Source: CAD feature listing. Evaluate the final solid. Frame: model axes, mm. Face numbers are marked on the shaded views. A direction names the side the tool comes from. Coordinates: 2 decimals unless noted, no trailing zeros. Order: outer loops, then holes, each group sorted by start corner. A loop starts at its lowest first (then second) coordinate and runs counter-clockwise, first axis right, second up. Notation, with made-up numbers: (67.5, -12.5) -> (105.5, -12.5) arc R25 cw to (105.5, -0.5) -> close; hole circle Ø8 at (26, -15.5). An arc over 180 degrees is marked (long way). Write item = value, one per line. Start each with the question number.
Item 1: Ray query, line 1 along Y through (x, z) = (-35, 22.25); line 2 along X through (y, z) = (20, 5.5); line 3 along X through (y, z) = (0, 11). Return the intervals inside material, ascending. Write a range as [from, to].
Item 2: Section query A-A (y = 0). Output: boundary loops of the cut face in (x, z), then the cut area to 3 significant figures.
Item 3: Contact query for flat-ended pins moving along their axis: pin 1 (1.5 mm diameter, centred on y = -18, z = 11.5, fed in from +X); pin 2 (3 mm diameter, centred on x = -39.5, z = 21.5, fed in from +Y); pin 3 (4 mm diameter, centred on x = -36.5, y = 28, fed in from -Z); pin 4 (2 mm diameter, centred on x = 32, z = 16, fed in from -Y). Output: stop coordinate, or through.
Item 4: Set-up query: the marked faces 1, 2 and 3. Return all of +Z, -Z, +X, -X, +Y, -Y with unobstructed straight access to the full face (end or side cutting, diameter ignored); none if empty.
Item 5: Section query C-C (y = -29). Output: boundary loops of the cut face in (x, z), then the cut area to 3 significant figures.
Item 6: Mould query, pull axis X, two halves, no side actions, for the marked faces 4, 5 and 6. Classes: released by +X, released by -X, zero draft, split by the parting line, or undercut.
Item 7: Section query B-B (y = -44). Output: boundary loops of the cut face in (x, z), then the cut area to 3 significant figures.
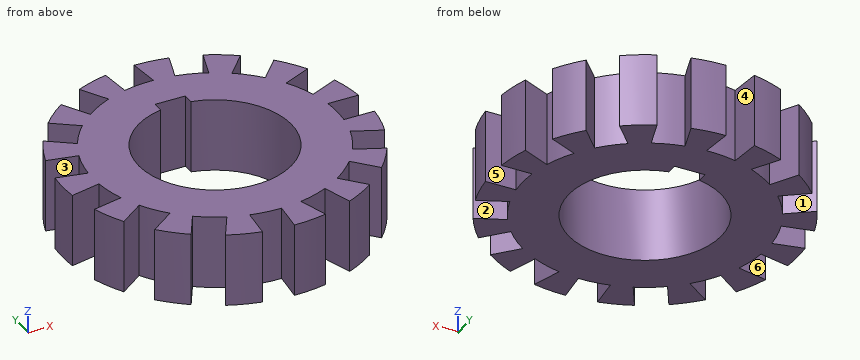
```python
from build123d import *

# Parameters (mm, degrees)
BOSS_EXTRUDE2_DEPTH = 24


with BuildPart() as part:
    # Sketch1 → Boss-Extrude2 (new body)
    with BuildSketch(Plane.XY):
        with BuildLine():
            Line((39.686269666, 5), (49.749371855, 5))
            ThreePointArc((49.749371855, 5), (48.907380037, 10.395584541), (47.481995894, 15.667165215))
            Line((47.481995894, 15.667165215), (38.2888946, 11.574132812))
            ThreePointArc((38.2888946, 11.574132812), (36.541818306, 16.269465723), (34.221528169, 20.709587388))
            Line((34.221528169, 20.709587388), (43.414629464, 24.802619792))
            ThreePointArc((43.414629464, 24.802619792), (40.450849719, 29.389262615), (37.004551483, 33.625335233))
            Line((37.004551483, 33.625335233), (30.271021813, 26.146992913))
            ThreePointArc((30.271021813, 26.146992913), (26.765224254, 29.725793019), (22.839573558, 32.838298977))
            Line((22.839573558, 32.838298977), (29.573103228, 40.316641297))
            ThreePointArc((29.573103228, 40.316641297), (25, 43.301270189), (20.128683944, 45.769379313))
            Line((20.128683944, 45.769379313), (17.019014352, 36.198800401))
            ThreePointArc((17.019014352, 36.198800401), (12.360679775, 38.042260652), (7.508449189, 39.288970345))
            Line((7.508449189, 39.288970345), (10.618118781, 48.859549256))
            ThreePointArc((10.618118781, 48.859549256), (5.226423163, 49.726094768), (-0.227615912, 49.999481907))
            Line((-0.227615912, 49.999481907), (0.824264696, 39.991506445))
            ThreePointArc((0.824264696, 39.991506445), (-4.181138531, 39.780875815), (-9.120954258, 38.946221812))
            Line((-9.120954258, 38.946221812), (-10.172834865, 48.954197275))
            ThreePointArc((-10.172834865, 48.954197275), (-15.450849719, 47.552825815), (-20.544558909, 45.584219849))
            Line((-20.544558909, 45.584219849), (-15.513007814, 36.869317712))
            ThreePointArc((-15.513007814, 36.869317712), (-20, 34.641016151), (-24.173261852, 31.869317712))
            Line((-24.173261852, 31.869317712), (-29.204812947, 40.584219849))
            ThreePointArc((-29.204812947, 40.584219849), (-33.456530318, 37.157241274), (-37.309161029, 33.287032059))
            Line((-37.309161029, 33.287032059), (-29.167940342, 27.372089))
            ThreePointArc((-29.167940342, 27.372089), (-32.360679775, 23.511410092), (-35.045792865, 19.281919056))
            Line((-35.045792865, 19.281919056), (-43.187013552, 25.196862116))
            ThreePointArc((-43.187013552, 25.196862116), (-45.677272882, 20.336832154), (-47.622670264, 15.234214023))
            Line((-47.622670264, 15.234214023), (-37.779471002, 13.141977432))
            ThreePointArc((-37.779471002, 13.141977432), (-39.125904029, 8.316467633), (-39.85858791, 3.360501425))
            Line((-39.85858791, 3.360501425), (-49.701787172, 5.452738016))
            ThreePointArc((-49.701787172, 5.452738016), (-50, 0), (-49.701787172, -5.452738016))
            Line((-49.701787172, -5.452738016), (-39.85858791, -3.360501425))
            ThreePointArc((-39.85858791, -3.360501425), (-39.125904029, -8.316467633), (-37.779471002, -13.141977432))
            Line((-37.779471002, -13.141977432), (-47.622670264, -15.234214023))
            ThreePointArc((-47.622670264, -15.234214023), (-45.677272882, -20.336832154), (-43.187013552, -25.196862116))
            Line((-43.187013552, -25.196862116), (-35.045792865, -19.281919056))
            ThreePointArc((-35.045792865, -19.281919056), (-32.360679775, -23.511410092), (-29.167940342, -27.372089))
            Line((-29.167940342, -27.372089), (-37.309161029, -33.287032059))
            ThreePointArc((-37.309161029, -33.287032059), (-33.456530318, -37.157241274), (-29.204812947, -40.584219849))
            Line((-29.204812947, -40.584219849), (-24.173261852, -31.869317712))
            ThreePointArc((-24.173261852, -31.869317712), (-20, -34.641016151), (-15.513007814, -36.869317712))
            Line((-15.513007814, -36.869317712), (-20.544558909, -45.584219849))
            ThreePointArc((-20.544558909, -45.584219849), (-15.450849719, -47.552825815), (-10.172834865, -48.954197275))
            Line((-10.172834865, -48.954197275), (-9.120954258, -38.946221812))
            ThreePointArc((-9.120954258, -38.946221812), (-4.181138531, -39.780875815), (0.824264696, -39.991506445))
            Line((0.824264696, -39.991506445), (-0.227615912, -49.999481907))
            ThreePointArc((-0.227615912, -49.999481907), (5.226423163, -49.726094768), (10.618118781, -48.859549256))
            Line((10.618118781, -48.859549256), (7.508449189, -39.288970345))
            ThreePointArc((7.508449189, -39.288970345), (12.360679775, -38.042260652), (17.019014352, -36.198800401))
            Line((17.019014352, -36.198800401), (20.128683944, -45.769379313))
            ThreePointArc((20.128683944, -45.769379313), (25, -43.301270189), (29.573103228, -40.316641297))
            Line((29.573103228, -40.316641297), (22.839573558, -32.838298977))
            ThreePointArc((22.839573558, -32.838298977), (26.765224254, -29.725793019), (30.271021813, -26.146992913))
            Line((30.271021813, -26.146992913), (37.004551483, -33.625335233))
            ThreePointArc((37.004551483, -33.625335233), (40.450849719, -29.389262615), (43.414629464, -24.802619792))
            Line((43.414629464, -24.802619792), (34.221528169, -20.709587388))
            ThreePointArc((34.221528169, -20.709587388), (36.541818306, -16.269465723), (38.2888946, -11.574132812))
            Line((38.2888946, -11.574132812), (47.481995894, -15.667165215))
            ThreePointArc((47.481995894, -15.667165215), (48.907380037, -10.395584541), (49.749371855, -5))
            Line((49.749371855, -5), (39.686269666, -5))
            ThreePointArc((39.686269666, -5), (40, 0), (39.686269666, 5))
        make_face()
        with BuildLine():
            Line((-5, 28), (5, 28))
            Line((5, 28), (5, 24.494897428))
            ThreePointArc((5, 24.494897428), (0, -25), (-5, 24.494897428))
            Line((-5, 24.494897428), (-5, 28))
        make_face(mode=Mode.SUBTRACT)
    extrude(amount=BOSS_EXTRUDE2_DEPTH)


solid = part.part
```
Computed:
q1.line_1 = [-35.71, -31.61], [-19.36, 19.36], [31.61, 35.71]
q1.line_2 = [-45.83, -36.03], [-34.64, -15], [15, 34.64]
q1.line_3 = [-50, -25], [25, 40]
q2.outline = (-50, 0) -> (-25, 0) -> (-25, 24) -> (-50, 24) -> close; (25, 0) -> (40, 0) -> (40, 24) -> (25, 24) -> close
q2.area = 960 mm^2
q3.pin_1 = 36.09
q3.pin_2 = 23.61
q3.pin_3 = through
q3.pin_4 = -29.18
q4.face_1 = +Z, -Z
q4.face_2 = +Z, -Z, +X
q4.face_3 = +Z, -Z, -X
q5.outline = (-31.41, 0) -> (27.55, 0) -> (27.55, 24) -> (-31.41, 24) -> close; (32.84, 0) -> (40.73, 0) -> (40.73, 24) -> (32.84, 24) -> close
q5.area = 1,600 mm^2
q6.face_4 = undercut
q6.face_5 = zero draft
q6.face_6 = released by -X
q7.outline = (-19.63, 0) -> (-9.65, 0) -> (-9.65, 24) -> (-19.63, 24) -> close; (0.4, 0) -> (9.04, 0) -> (9.04, 24) -> (0.4, 24) -> close; (19.55, 0) -> (23.75, 0) -> (23.75, 24) -> (19.55, 24) -> close
q7.area = 547 mm^2
